from build123d import *

# Parameters (mm, degrees)
BOSS_EXTRUDE1_DEPTH = 15
SKETCH2_R           = 12.5
BOSS_EXTRUDE2_DEPTH = 5
SKETCH3_R           = 5
CUT_EXTRUDE1_DEPTH  = 37.514837167
CHAMFER1_SIZE       = 5
SKETCH4_R           = 12.5
CUT_EXTRUDE2_DEPTH  = 5


with BuildPart() as part:
    # Sketch1 → Boss-Extrude1 (new body)
    with BuildSketch(Plane(origin=(0, 0, 0), x_dir=(1, 0, 0), z_dir=(0, 1, 0))):
        Polygon((11.547005384, 20), (-11.547005384, 20), (-23.094010768, 0), (-11.547005384, -20), (11.547005384, -20), (23.094010768, 0), align=None)
    extrude(amount=BOSS_EXTRUDE1_DEPTH)

    # Sketch2 → Boss-Extrude2 (add)
    with BuildSketch(Plane(origin=(0, 15, 0), x_dir=(1, 0, 0), z_dir=(0, 1, 0))):
        with Locations(Location((0, 0, 0), (0, 0, 270))):
            Circle(SKETCH2_R)
    extrude(amount=BOSS_EXTRUDE2_DEPTH)

    # Sketch3 → Cut-Extrude1 (cut, through all)
    with BuildSketch(Plane(origin=(0, 20, 0), x_dir=(1, 0, 0), z_dir=(0, 1, 0))):
        with Locations(Location((0, 0, 0), (0, 0, 270))):
            Circle(SKETCH3_R)
    extrude(amount=-CUT_EXTRUDE1_DEPTH, mode=Mode.SUBTRACT)

    # Chamfer1
    chamfer1_edges = [part.edges().sort_by_distance(p)[0] for p in [
        (0, 20, -12.5),
    ]]
    chamfer(chamfer1_edges, length=CHAMFER1_SIZE - 0.0001)  # a hair under: the kernel refuses the full size

    # Sketch4 → Cut-Extrude2 (cut)
    with BuildSketch(Plane.XZ):
        with Locations(Location((0, 0, 0), (0, 0, 270))):
            Circle(SKETCH4_R)
    extrude(amount=-CUT_EXTRUDE2_DEPTH, mode=Mode.SUBTRACT)


solid = part.part
Source: CAD feature listing. Evaluate the final solid. Frame: model axes, mm. A direction names the side the tool comes from. Give positions to 0.01 mm unless a question says otherwise; leave off trailing zeros. Order: outer loops, then holes, each group sorted by start corner. A loop starts at its lowest first (then second) coordinate and runs counter-clockwise, first axis right, second up. Notation, with made-up numbers: (86, 33.25) -> (129, 33.25) arc R24 cw to (129, 48.25) -> close; hole circle Ø8 at (43.5, -3). An arc over 180 degrees is marked (long way). Use a Markdown table: item, result.
1) Contact query for flat-ended pins moving along their axis: P1, Ø15, axis at x = 0, z = 0, coming from the -Y side; P2, Ø10, axis at x = 11, z = -16, coming from the +Y side; P3, Ø2, axis at y = 8.5, z = 3.5, coming from the -X side. Output: stop coordinate, or through.
Answer list:
| item | result |
|---|---|
| P1 | y = 5 |
| P2 | y = 15 |
| P3 | x = -21.65 |
2) Section query D-D, the plane z = -14. Return the cut outline in (x, y).
Answer list:
| item | result |
|---|---|
| outline | (-15.01, 0) -> (15.01, 0) -> (15.01, 15) -> (-15.01, 15) -> close |
3) Mould query, pull axis Z, two halves, no side actions, for faces 1 (the cylindrical face through (3.755, 2.465, -11.923)), 2 (the flat face through (17.24, 7.4, 10.14)), 3 (the flat face through (0, 7, -20)), 4 (the flat face through (-5.4, 5, 0.2)). Classes: +Z half, -Z half, draft (parallel to the pull), parting line (faces both ways), or undercut.
Answer list:
| item | result |
|---|---|
| face 1 | undercut |
| face 2 | +Z half |
| face 3 | -Z half |
| face 4 | undercut |
4) Reachability of faces 5 (the flat face through (10, 15, -9)), 6 (the cylindrical face through (-4.88, 12.6, -1.08)) from +Z, -Z, +X, -X, +Y, -Y: full face, straight path, thin tool, end or side. Return the list, or none.
Answer list:
| item | result |
|---|---|
| face 5 | +Y |
| face 6 | +Y, -Y |
5) Ray query, line 1 along X through (y, z) = (1.1, 0); line 2 along X through (y, z) = (10, 0); line 3 along Z through (x, y) = (-0.5, 1). Return the intervals inside material, ascending. Write a range as [from, to].
Answer list:
| item | result |
|---|---|
| line 1 | [-23.09, -12.5], [12.5, 23.09] |
| line 2 | [-23.09, -5], [5, 23.09] |
| line 3 | [-20, -12.49], [12.49, 20] |
6) Section query A-A, the plane y = 8.5. Return the cut outline in (x, z).
Answer list:
| item | result |
|---|---|
| outline | (-23.09, 0) -> (-11.55, -20) -> (11.55, -20) -> (23.09, 0) -> (11.55, 20) -> (-11.55, 20) -> close; hole circle Ø10 at (0, 0) |
7) Section query C-C, the plane x = -15. Return the cut outline in (y, z).
Answer list:
| item | result |
|---|---|
| outline | (0, -14.02) -> (15, -14.02) -> (15, 14.02) -> (0, 14.02) -> close |
